from build123d import *

# Parameters (mm, degrees)
SKETCH1_W           = 1700
SKETCH1_H           = 500
BOSS_EXTRUDE1_DEPTH = 500
SHELL1_T            = -4
SKETCH2_W           = 100
SKETCH2_H           = 100
BOSS_EXTRUDE2_DEPTH = 1700


with BuildPart() as part:
    # Sketch1 → Boss-Extrude1 (new body)
    with BuildSketch(Plane.XY):
        with Locations((850, 250)):
            Rectangle(SKETCH1_W, SKETCH1_H)
    extrude(amount=BOSS_EXTRUDE1_DEPTH)

    # Shell1
    shell1_openings = [part.faces().sort_by_distance(p)[0] for p in [
        (850, 500, 250),
    ]]
    offset(amount=SHELL1_T, openings=shell1_openings, kind=Kind.INTERSECTION)

    # Sketch2 → Boss-Extrude2 (add)
    with BuildSketch(Plane(origin=(1700, 0, 0), x_dir=(0, 0, -1), z_dir=(1, 0, 0))):
        with Locations((-250, 550)):
            Rectangle(SKETCH2_W, SKETCH2_H)
    extrude(amount=-BOSS_EXTRUDE2_DEPTH)


solid = part.part
Geometry: final body of the model. Coordinates: model frame, mm. A direction names the side the tool comes from. Give positions to 0.01 mm unless a question says otherwise; leave off trailing zeros. Loops run counter-clockwise (first coordinate to the right, second up) from the corner with the lowest first, then second, coordinate; pieces in that order, holes last. Notation, with made-up numbers: M -24,87.25 L -9,87.25 A3 ccw -9,92.25 Z; hole C 51.5,80.25 d3. An arc over 180 degrees is marked long. Put each result on its own line as item: value. Start each with the question number.
1) Pull-direction query (Y, two-part tool) for faces 1 (the flat face through (838, 254, 0)), 2 (the flat face through (846, 500, 3)), 3 (the flat face through (838, 0, 246)), 4 (the flat face through (862, 500, 251)); classes: pulls with the +Y half, pulls with the -Y half, needs draft (parallel to the pull), parting line crosses it, or undercut.
2) Access query for faces 5 (the flat face through (862, 549, 300)), 6 (the flat face through (838, 255, 496)), 7 (the flat face through (862, 549, 200)). Directions: +Z, -Z, +X, -X, +Y, -Y. A direction counts if a zero-diameter tool reaches every point of the face in a straight line with its end or side. Return the directions, or none.
3) Ray query, line 1 along Y through (x, z) = (509.5, 213); line 2 along X through (y, z) = (339, 381.5); line 3 along Z through (x, y) = (410.5, 217). Return the intervals inside material, ascending.
4) Contact query for a flat-ended pin moving along its axis: pin 1 (1.5 mm diameter, centred on x = 847, z = 303, fed in from +Y). Output: stop coordinate, or through.
5) Cut plane A-A (x = 825). Output: boundary loops of the cut face in (y, z), then the cut area to 3 significant figures.
6) Cut plane D-D (z = 126.5). Output: boundary loops of the cut face in (x, y).
7) Cut plane C-C (y = 140). Output: boundary loops of the cut face in (x, z).
8) Cut plane B-B (z = 251.5). Output: boundary loops of the cut face in (x, y), then the cut area to 3 significant figures.
Verdict:
1. face 1: needs draft
1. face 2: pulls with the +Y half
1. face 3: pulls with the -Y half
1. face 4: undercut
2. face 5: +Z, +X, -X, +Y
2. face 6: +Y
2. face 7: -Z, +X, -X, +Y
3. line 1: 0 to 4, 500 to 600
3. line 2: 0 to 4, 1696 to 1700
3. line 3: 0 to 4, 496 to 500
4. pin 1: y = 4
5. outline: M 0,0 L 500,0 L 500,4 L 4,4 L 4,496 L 500,496 L 500,500 L 0,500 Z; M 500,200 L 600,200 L 600,300 L 500,300 Z
5. area: 16,000 mm2
6. outline: M 0,0 L 1700,0 L 1700,500 L 1696,500 L 1696,4 L 4,4 L 4,500 L 0,500 Z
7. outline: M 0,0 L 1700,0 L 1700,500 L 0,500 Z; hole M 4,4 L 1696,4 L 1696,496 L 4,496 Z
8. outline: M 0,0 L 1700,0 L 1700,600 L 0,600 Z; hole M 4,4 L 1696,4 L 1696,500 L 4,500 Z
8. area: 181,000 mm2
